from build123d import *

# Parameters (mm, degrees)
BOSS_EXTRUDE1_DEPTH = 1
SKETCH2_W           = 12
SKETCH2_H           = 4
BOSS_EXTRUDE2_DEPTH = 1
SKETCH3_R           = 1
SKETCH3_R_2         = 0.426779722
CUT_EXTRUDE1_DEPTH  = 16.652475842
BOSS_EXTRUDE3_DEPTH = 2
SKETCH5_W           = 8.547335384
SKETCH5_H           = 5.323692461
BOSS_EXTRUDE4_DEPTH = 1


with BuildPart() as part:
    # Sketch1 → Boss-Extrude1 (new body)
    with BuildSketch(Plane(origin=(0, 0, 0), x_dir=(1, 0, 0), z_dir=(0, 1, 0))):
        with BuildLine():
            Line((-6, 12), (6, 12))
            ThreePointArc((6, 12), (10, 8), (6, 4))
            Line((6, 4), (-6, 4))
            ThreePointArc((-6, 4), (-10, 8), (-6, 12))
        make_face()
    extrude(amount=BOSS_EXTRUDE1_DEPTH)

    # Sketch2 → Boss-Extrude2 (add)
    with BuildSketch(Plane.XZ):
        with Locations((0, -2)):
            Rectangle(SKETCH2_W, SKETCH2_H)
    extrude(amount=-BOSS_EXTRUDE2_DEPTH)

    # Sketch3 → Cut-Extrude1 (cut, through all)
    with BuildSketch(Plane(origin=(0, 1, 0), x_dir=(1, 0, 0), z_dir=(0, 1, 0))):
        with Locations(Location((8, 8, 0), (0, 0, 270))):
            Circle(SKETCH3_R)
        with Locations(Location((-8, 8, 0), (0, 0, 270))):
            Circle(SKETCH3_R)
        with Locations(Location((-4.895656887, 0.783316432, 0), (0, 0, 270))):
            Circle(SKETCH3_R_2)
        with Locations(Location((-3.145656887, 0.783316432, 0), (0, 0, 270))):
            Circle(SKETCH3_R_2)
        with Locations(Location((-1.395656887, 0.783316432, 0), (0, 0, 270))):
            Circle(SKETCH3_R_2)
        with Locations(Location((0.354343113, 0.783316432, 0), (0, 0, 270))):
            Circle(SKETCH3_R_2)
        with Locations(Location((2.104343113, 0.783316432, 0), (0, 0, 270))):
            Circle(SKETCH3_R_2)
        with Locations(Location((3.854343113, 0.783316432, 0), (0, 0, 270))):
            Circle(SKETCH3_R_2)
    extrude(amount=-CUT_EXTRUDE1_DEPTH, mode=Mode.SUBTRACT)

    # Sketch4 → Boss-Extrude3 (add)
    with BuildSketch(Plane(origin=(0, 1, 0), x_dir=(1, 0, 0), z_dir=(0, 1, 0))):
        with BuildLine():
            Line((-2.294003159, 10.093090184), (2.294003159, 10.093090184))
            ThreePointArc((2.294003159, 10.093090184), (4.688327155, 7.698766187), (2.294003159, 5.304442191))
            Line((2.294003159, 5.304442191), (-2.294003159, 5.304442191))
            ThreePointArc((-2.294003159, 5.304442191), (-4.688327155, 7.698766187), (-2.294003159, 10.093090184))
        make_face()
    extrude(amount=BOSS_EXTRUDE3_DEPTH)

    # Sketch5 → Boss-Extrude4 (add)
    with BuildSketch(Plane.XZ):
        with Locations((-0.127073061, -6.949703932)):
            Rectangle(SKETCH5_W, SKETCH5_H)
    extrude(amount=BOSS_EXTRUDE4_DEPTH)


solid = part.part
Here's how the part is built. I have some questions about the finished solid (model axes, mm). A direction names the side the tool comes from. Coordinates: 2 decimals unless noted, no trailing zeros. Write each loop counter-clockwise with the first axis right and the second up, starting at its lowest first coordinate (ties: lowest second). Pieces come first, ordered by that corner, then holes.
1) If we section it at C-C (y = 2.5): List the corners of the cut face in (x, z) for me.
Filled in:
outline: (-2.29, -10.09) - (2.29, -10.09) arc R2.39 ccw to (2.29, -5.3) - (-2.29, -5.3) arc R2.39 ccw to start
2) If we section it at B-B (x = -8): List the corners of the cut face in (y, z) for me.
Filled in:
outline: (0, -11.46) - (1, -11.46) - (1, -9) - (0, -9) - close; (0, -7) - (1, -7) - (1, -4.54) - (0, -4.54) - close
3) If we section it at D-D (z = -2): List the corners of the cut face in (x, y) for me.
Filled in:
outline: (-6, 0) - (6, 0) - (6, 1) - (-6, 1) - close
4) I'm going to push flat-ended pins straight in: pin 1 (2.5 mm diameter, centred on x = -8, z = -8, fed in from -Y); pin 2 (0.5 mm diameter, centred on y = -0.5, z = -6.5, fed in from -X); pin 3 (1.8 mm diameter, centred on x = 8, z = -8, fed in from -Y); pin 4 (2 mm diameter, centred on y = 1, z = -1.5, fed in from +X). Where does each tip first touch, or does it pass through?
Filled in:
pin 1: stops at y = 0
pin 2: stops at x = -4.4
pin 3: passes through
pin 4: stops at x = 6
5) If we section it at A-A (z = -8): List the corners of the cut face in (x, y) for me.
Filled in:
outline: (-10, 0) - (-9, 0) - (-9, 1) - (-10, 1) - close; (-7, 0) - (-4.4, 0) - (-4.4, -1) - (4.15, -1) - (4.15, 0) - (7, 0) - (7, 1) - (4.67, 1) - (4.67, 3) - (-4.67, 3) - (-4.67, 1) - (-7, 1) - close; (9, 0) - (10, 0) - (10, 1) - (9, 1) - close
6) Which directions (+Z, -Z, +X, -X, +Y, -Y) give clear straight access to the entire face, cutting with the end or side of a thin tool? Please do faces 1 (the face through (0, 2, -5.304)), 2 (the face through (0, 1, -5)), 3 (the face through (-0.2, -0.5, -4.288)).
Filled in:
face 1: +Z, +X, -X, +Y
face 2: +Y
face 3: +Z, +X, -X, -Y
7) If I drill on line 1 (X direction, y = 0.65, z = -8); line 2 (X direction, y = 0.2, z = -1.75); line 3 (Y direction, x = -3.5, z = -5.25), over which ranges is the centre line in solid material (lowest first)?
Filled in:
line 1: x = -10 to -9, -7 to 7, 9 to 10
line 2: x = -6 to 6
line 3: y = -1 to 1
8) Thinking about a two-plate mould opening in X: for faces 4 (the face through (-4.473, 0.507, -0.839)), 5 (the face through (4.688, 1.986, -7.751)), 6 (the face through (0, 0, -10)), which applies, +X half, -X half, draft (parallel to the pull), parting line (faces both ways), or undercut?
Filled in:
face 4: undercut
face 5: +X half
face 6: draft
